Build history of the part. All positions in model axes, mm. Give positions to 0.01 mm unless a question says otherwise; leave off trailing zeros. Loops run counter-clockwise (first coordinate to the right, second up) from the corner with the lowest first, then second, coordinate; pieces in that order, holes last.
1) Two-plate mould, pull along Z, no slides. Class faces 1 (the flat face through (22.109, 2, 0)), 2 (the cylindrical face through (-18.83, 1.97, -1.08)), 3 (the cylindrical face through (21.207, 2.028, -3.026)): +Z half, -Z half, draft (parallel to the pull), parting line (faces both ways), or undercut.
2) Band-saw the part on D-D on z = -3.25. List the corners of the cut face in (x, y).
3) Band-saw the part on A-A on x = -17.65. List the corners of the cut face in (y, z), then the cut area to 3 significant figures.
4) Wall check: line 1 (X direction, y = 0.8, z = 0); line 2 (Z direction, x = 17.65, y = 2.15); line 3 (X direction, y = 3.5, z = -1). Give the ranges that are in metal, low to high.
5) Flat gauge pins, fed straight in: P1, Ø1, axis at y = 3.5, z = 2, coming from the +X side; P2, Ø3, axis at x = -17.65, z = 0, coming from the -Y side. Where does each tip first touch, or does it go through?
6) Band-saw the part on C-C on y = 1.1. List the corners of the cut face in (x, z).
7) Band-saw the part on B-B on z = 0. List the corners of the cut face in (x, y), then the cut area to 3 significant figures.
```python
from build123d import *

# Parameters (mm, degrees)
SKETCH_1_W      = 44.217702276
SKETCH_1_H      = 7.762687128
SKETCH_1_R      = 1.6
EXTRUDE_1_DEPTH = 4
FILLET_1_R      = 3


with BuildPart() as part:
    # 草图1 → 凸台-拉伸1 (new body)
    with BuildSketch(Plane(origin=(0, 0, 0), x_dir=(1, 0, 0), z_dir=(0, 1, 0))):
        Rectangle(SKETCH_1_W, SKETCH_1_H)
        with Locations((-17.65, 0)):
            Circle(SKETCH_1_R, mode=Mode.SUBTRACT)
        with Locations((17.65, 0)):
            Circle(SKETCH_1_R, mode=Mode.SUBTRACT)
    extrude(amount=EXTRUDE_1_DEPTH)

    # 圆角1
    fillet_1_edges = [part.edges().sort_by_distance(p)[0] for p in [
        (-22.108851138, 2, -3.881343564),
        (22.108851138, 2, -3.881343564),
        (22.108851138, 2, 3.881343564),
        (-22.108851138, 2, 3.881343564),
    ]]
    fillet(fillet_1_edges, radius=FILLET_1_R)


solid = part.part
```
Findings below:
1. face 1: draft
1. face 2: undercut
1. face 3: -Z half
2. outline: (-20.95, 0) - (20.95, 0) - (20.95, 4) - (-20.95, 4) - close
3. outline: (0, -3.88) - (4, -3.88) - (4, -1.6) - (0, -1.6) - close; (0, 1.6) - (4, 1.6) - (4, 3.88) - (0, 3.88) - close
3. area: 18.3 mm2
4. line 1: x = -22.11 to -19.25, -16.05 to 16.05, 19.25 to 22.11
4. line 2: z = -3.88 to -1.6, 1.6 to 3.88
4. line 3: x = -22.11 to -18.9, -16.4 to 16.4, 18.9 to 22.11
5. P1: stops at x = 22.04
5. P2: passes through
6. outline: (-22.11, -0.88) arc R3 ccw to (-19.11, -3.88) - (19.11, -3.88) arc R3 ccw to (22.11, -0.88) - (22.11, 0.88) arc R3 ccw to (19.11, 3.88) - (-19.11, 3.88) arc R3 ccw to (-22.11, 0.88) - close; hole circle Ø3.2 at (-17.65, 0); hole circle Ø3.2 at (17.65, 0)
7. outline: (-22.11, 0) - (-19.25, 0) - (-19.25, 4) - (-22.11, 4) - close; (-16.05, 0) - (16.05, 0) - (16.05, 4) - (-16.05, 4) - close; (19.25, 0) - (22.11, 0) - (22.11, 4) - (19.25, 4) - close
7. area: 151 mm2
